```python
from build123d import *

# Parameters (mm, degrees)
SKETCH1_R           = 7.9375
SKETCH1_R_2         = 3.175
BOSS_EXTRUDE1_DEPTH = 1.5875
SKETCH2_R           = 3.96875
SKETCH2_R_2         = 3.175
BOSS_EXTRUDE2_DEPTH = 3.175
SKETCH3_R           = 3.937
SKETCH3_R_2         = 3.175
BOSS_EXTRUDE3_DEPTH = 0.79375


with BuildPart() as part:
    # Sketch1 → Boss-Extrude1 (new body)
    with BuildSketch(Plane(origin=(0, 0, 0), x_dir=(1, 0, 0), z_dir=(0, 1, 0))):
        Circle(SKETCH1_R)
        Circle(SKETCH1_R_2, mode=Mode.SUBTRACT)
    extrude(amount=BOSS_EXTRUDE1_DEPTH)

    # Sketch2 → Boss-Extrude2 (add)
    with BuildSketch(Plane(origin=(0, 1.5875, 0), x_dir=(1, 0, 0), z_dir=(0, 1, 0))):
        Circle(SKETCH2_R)
        Circle(SKETCH2_R_2, mode=Mode.SUBTRACT)
    extrude(amount=BOSS_EXTRUDE2_DEPTH)

    # Sketch3 → Boss-Extrude3 (add)
    with BuildSketch(Plane.XZ):
        Circle(SKETCH3_R)
        Circle(SKETCH3_R_2, mode=Mode.SUBTRACT)
    extrude(amount=BOSS_EXTRUDE3_DEPTH)


solid = part.part
```
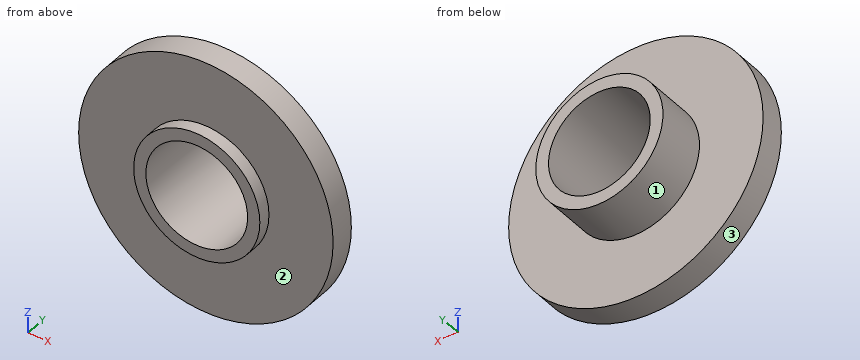
Geometry check sheet. Reference: the model listing, model coordinates, mm. Face numbers are marked on the shaded views. A direction names the side the tool comes from. Give positions to 0.01 mm unless a question says otherwise; leave off trailing zeros. Loops run counter-clockwise (first coordinate to the right, second up) from the corner with the lowest first, then second, coordinate; pieces in that order, holes last. Notation, with made-up numbers: (-17, 73.5) - (-1, 73.5) arc R23 cw to (-1, 96.5) - close; hole circle Ø6 at (-32, 25). An arc over 180 degrees is marked (long way). Use CSV: the item, a comma, the result in double quotes. Start each with the question number.
Q1. Section check B-B, the plane z = 0. Record the cut outline in (x, y) (1 decimal).
Q2. Access from +Z, -Z, +X, -X, +Y, -Y to the whole of each face (thin tool, end or side, straight path). Record for the marked faces 1, 2 and 3.
Q3. Go/stop test with flat-tipped pins: pin 1 Ø1 at (y, z) = (1.5, 2) entering from -X; pin 2 Ø2 at (x, z) = (-6.5, 2) entering from +Y; pin 3 Ø2 at (x, y) = (-2.5, 2) entering from +Z. Record where each tip stops, or that it passes through.
Q4. Section check A-A, the plane x = 0. Record the cut outline in (y, z) (1 decimal), and give its area (3 significant figures).
Q5. Scan lines: probe 1 along X at (y, z) = (1.55, 0) (1 decimal); probe 2 along X at (y, z) = (1.9, 0) (3 decimals); probe 3 along Y at (x, z) = (-4, -0.5). Record each from-to range of solid material in increasing order. Write a range as from..to.
Q6. Section check D-D, the plane x = -6.5. Record the cut outline in (y, z).
Findings below:
1,outline,"(-7.9, 0) - (-3.9, 0) - (-3.9, -0.8) - (-3.2, -0.8) - (-3.2, 4.8) - (-4, 4.8) - (-4, 1.6) - (-7.9, 1.6) - close; (3.2, -0.8) - (3.9, -0.8) - (3.9, 0) - (7.9, 0) - (7.9, 1.6) - (4, 1.6) - (4, 4.8) - (3.2, 4.8) - close"
2,face 1,"+Y"
2,face 2,"-Y"
2,face 3,"+Y, -Y"
3,pin 1,"stops at x = -7.79"
3,pin 2,"stops at y = 1.59"
3,pin 3,"stops at z = 7.78"
4,outline,"(-0.8, -3.9) - (0, -3.9) - (0, -7.9) - (1.6, -7.9) - (1.6, -4) - (4.8, -4) - (4.8, -3.2) - (-0.8, -3.2) - close; (-0.8, 3.2) - (4.8, 3.2) - (4.8, 4) - (1.6, 4) - (1.6, 7.9) - (0, 7.9) - (0, 3.9) - (-0.8, 3.9) - close"
4,area,"21.4 mm^2"
5,probe 1,"x = -7.9..-3.2, 3.2..7.9"
5,probe 2,"x = -3.969..-3.175, 3.175..3.969"
5,probe 3,"y = 0..1.59"
6,outline,"(0, -4.56) - (1.59, -4.56) - (1.59, 4.56) - (0, 4.56) - close"
